Can you work these out from the model? Positions are in its coordinate system, mm. Face numbers are marked on the shaded views. A direction names the side the tool comes from. Coordinates: 2 decimals unless noted, no trailing zeros. Order: outer loops, then holes, each group sorted by start corner. A loop starts at its lowest first (then second) coordinate and runs counter-clockwise, first axis right, second up. Notation, with made-up numbers: (46, 4.5) -> (63, 4.5) arc R26 cw to (63, 26.5) -> close; hole circle Ø8 at (19, 56.5). An arc over 180 degrees is marked (long way). Use a Markdown table: item, result. Add a question column.
1. For the marked faces 1, 2 and 3, which set-ups out of +Z, -Z, +X, -X, +Y, -Y let a thin tool reach every point of the face, with its end or its side?
2. For pin 1 Ø2 at (x, y) = (10.5, 2) entering from -Z; pin 2 Ø4 at (x, z) = (23, 1) entering from +Y; pin 3 Ø4.5 at (x, z) = (-17.5, 3) entering from +Y; pin 4 Ø2.5 at (x, y) = (-21.5, -20.5) entering from +Z, each with a flat end and sliding along its axis, tell me the tip position at first contact or that it passes through.
3. Suppose I cut it at A-A, the plane x = 16. List the corners of the cut face in (y, z) for me.
4. If I drill on line 1 along Y through (x, z) = (-25.5, 4.5); line 2 along Y through (x, z) = (-15, 3.75); line 3 along X through (y, z) = (27, 6) (3 decimals), over which ranges is the centre line in solid material (lowest first)? Write a range as from..to.
5. We'd pull the mould along Y, two halves only. Please class the marked faces 4, 5 and 6: pulls with the +Y half, pulls with the -Y half, needs draft (parallel to the pull), parting line crosses it, or undercut.
6. Suppose I cut it at B-B, the plane z = 6.75. State how many separate pieces and enclosed holes the cut face has, then the cut area to 3 significant figures.
```python
from build123d import *

# Parameters (mm, degrees)
SKETCH_1_W          = 70
SKETCH_1_H          = 80
EXTRUDE_1_DEPTH     = 8
SKETCH_11_R         = 3
CUT_EXTRUDE_4_DEPTH = 15
SKETCH_13_R         = 4.55
CUT_EXTRUDE_6_DEPTH = 6
SKETCH_14_R         = 3
CUT_EXTRUDE_7_DEPTH = 16
CUT_EXTRUDE_8_DEPTH = 5.4
FILLET_1_R          = 20


with BuildPart() as part:
    # 草图1 → 凸台-拉伸1 (new body)
    with BuildSketch(Plane.XY):
        Rectangle(SKETCH_1_W, SKETCH_1_H)
    extrude(amount=EXTRUDE_1_DEPTH)

    # 草图11 → 切除-拉伸4 (cut)
    with BuildSketch(Plane.XY):
        with Locations((-22.273863607, 26.273863607)):
            Circle(SKETCH_11_R)
        with Locations((22.273863607, 26.273863607)):
            Circle(SKETCH_11_R)
        with Locations((22.273863607, -18.273863607)):
            Circle(SKETCH_11_R)
        with Locations((-22.273863607, -18.273863607)):
            Circle(SKETCH_11_R)
    extrude(amount=CUT_EXTRUDE_4_DEPTH, mode=Mode.SUBTRACT)

    # 草图13 → 切除-拉伸6 (cut)
    with BuildSketch(Plane.XY.offset(8)):
        with Locations((-22.273863607, 26.273863607)):
            Circle(SKETCH_13_R)
        with Locations((-22.273863607, -18.273863607)):
            Circle(SKETCH_13_R)
        with Locations(Location((22.273863607, -18.273863607, 0), (0, 0, 180))):
            Circle(SKETCH_13_R)
        with Locations(Location((22.273863607, 26.273863607, 0), (0, 0, 180))):
            Circle(SKETCH_13_R)
    extrude(amount=-CUT_EXTRUDE_6_DEPTH, mode=Mode.SUBTRACT)

    # 草图14 → 切除-拉伸7 (cut)
    with BuildSketch(Plane.XY.offset(8)):
        with Locations((-17.56, 5.56)):
            Circle(SKETCH_14_R)
        with Locations((17.56, 5.56)):
            Circle(SKETCH_14_R)
        with Locations((17.56, -29.56)):
            Circle(SKETCH_14_R)
        with Locations((-17.56, -29.56)):
            Circle(SKETCH_14_R)
    extrude(amount=-CUT_EXTRUDE_7_DEPTH, mode=Mode.SUBTRACT)

    # 草图15 → 切除-拉伸8 (cut)
    with BuildSketch(Plane(origin=(0, 0, 0), x_dir=(-1, 0, 0), z_dir=(0, 0, -1))):
        Polygon((-14.713663173, 0.63), (-11.867326346, 5.56), (-14.713663173, 10.49), (-20.406336827, 10.49), (-23.252673654, 5.56), (-20.406336827, 0.63), align=None)
        Polygon((-14.713663173, -34.49), (-11.867326346, -29.56), (-14.713663173, -24.63), (-20.406336827, -24.63), (-23.252673654, -29.56), (-20.406336827, -34.49), align=None)
        Polygon((20.406336827, -34.49), (14.713663173, -34.49), (11.867326346, -29.56), (14.713663173, -24.63), (20.406336827, -24.63), (23.252673654, -29.56), align=None)
        Polygon((20.406336827, 0.63), (14.713663173, 0.63), (11.867326346, 5.56), (14.713663173, 10.49), (20.406336827, 10.49), (23.252673654, 5.56), align=None)
    extrude(amount=-CUT_EXTRUDE_8_DEPTH, mode=Mode.SUBTRACT)

    # 圆角1
    fillet_1_edges = [part.edges().sort_by_distance(p)[0] for p in [
        (-35, 40, 4),
        (35, 40, 4),
        (35, -40, 4),
        (-35, -40, 4),
    ]]
    fillet(fillet_1_edges, radius=FILLET_1_R)


solid = part.part
```
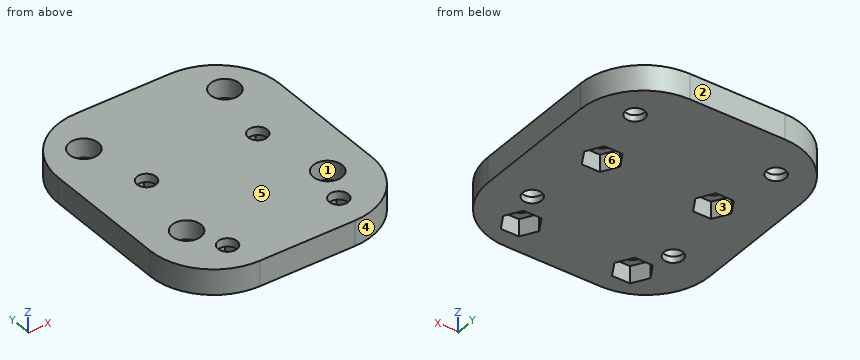
Worked out:
| question | item | result |
|---|---|---|
| 1 | face 1 | +Z |
| 1 | face 2 | +Z, -Z, +X, -X, +Y |
| 1 | face 3 | -Z |
| 2 | pin 1 | stops at z = 0 |
| 2 | pin 2 | stops at y = 39.08 |
| 2 | pin 3 | stops at y = 40 |
| 2 | pin 4 | stops at z = 2 |
| 3 | outline | (-39.97, 0) -> (-34.49, 0) -> (-34.49, 5.4) -> (-32.12, 5.4) -> (-32.12, 8) -> (-39.97, 8) -> close; (-27, 5.4) -> (-24.63, 5.4) -> (-24.63, 0) -> (0.63, 0) -> (0.63, 5.4) -> (3, 5.4) -> (3, 8) -> (-27, 8) -> close; (8.12, 5.4) -> (10.49, 5.4) -> (10.49, 0) -> (39.97, 0) -> (39.97, 8) -> (8.12, 8) -> close |
| 4 | line 1 | y = -37.02..-21.48, -15.07..23.07, 29.48..37.02 |
| 4 | line 2 | y = -40..-34.49, -24.63..0.63, 10.49..40 |
| 4 | line 3 | x = -33.735..-26.766, -17.782..17.782, 26.766..33.735 |
| 5 | face 4 | pulls with the -Y half |
| 5 | face 5 | needs draft |
| 5 | face 6 | undercut |
| 6 | separate pieces | 1 |
| 6 | enclosed holes | 8 |
| 6 | area | 4,880 mm² |
